from build123d import *

# Parameters (mm, degrees)
SKETCH7_R           = 1.5
SKETCH7_R_2         = 3.5
SKETCH7_R_3         = 1
BOSS_EXTRUDE1_DEPTH = 3.5
FILLET8_R           = 10
FILLET14_R          = 1
FILLET15_R          = 1
FILLET16_R          = 1


with BuildPart() as part:
    # Sketch7 → Boss-Extrude1 (new body)
    with BuildSketch(Plane.XY):
        with BuildLine():
            Line((81.96877708, 8.838834765), (95.403805922, -4.596194078))
            ThreePointArc((95.403805922, -4.596194078), (104.596194078, -4.596194078), (104.596194078, 4.596194078))
            Line((104.596194078, 4.596194078), (91.161165235, 18.03122292))
            Line((91.161165235, 18.03122292), (93.636038969, 20.506096654))
            Line((93.636038969, 20.506096654), (44.142135624, 70))
            Line((44.142135624, 70), (6, 70))
            Line((6, 70), (3.453220204, 85.420324662))
            ThreePointArc((3.453220204, 85.420324662), (0, 88.35), (-3.453220204, 85.420324662))
            Line((-3.453220204, 85.420324662), (-6, 70))
            Line((-6, 70), (-44.142135624, 70))
            Line((-44.142135624, 70), (-63.587572106, 50.554563517))
            Line((-63.587572106, 50.554563517), (-49.445436483, 36.412427894))
            Line((-49.445436483, 36.412427894), (-35.857864376, 50))
            Line((-35.857864376, 50), (35.857864376, 50))
            Line((35.857864376, 50), (79.493903346, 6.363961031))
            Line((79.493903346, 6.363961031), (81.96877708, 8.838834765))
        make_face()
        with Locations((0, 84.85)):
            Circle(SKETCH7_R, mode=Mode.SUBTRACT)
        with Locations((0, 60)):
            Circle(SKETCH7_R, mode=Mode.SUBTRACT)
        with Locations((100, 0)):
            Circle(SKETCH7_R_2, mode=Mode.SUBTRACT)
        with Locations((86.564971157, 20.506096654)):
            Circle(SKETCH7_R_3, mode=Mode.SUBTRACT)
        with Locations((79.493903346, 13.435028843)):
            Circle(SKETCH7_R_3, mode=Mode.SUBTRACT)
        with Locations((-50, 50)):
            Circle(SKETCH7_R, mode=Mode.SUBTRACT)
    extrude(amount=BOSS_EXTRUDE1_DEPTH)

    # Fillet8
    fillet8_edges = [part.edges().sort_by_distance(p)[0] for p in [
        (-44.142135624, 70, 1.75),
        (44.142135624, 70, 1.75),
    ]]
    fillet(fillet8_edges, radius=FILLET8_R)

    # Fillet14
    fillet14_edges = [part.edges().sort_by_distance(p)[0] for p in [
        (93.636038969, 20.506096654, 1.75),
        (91.161165235, 18.03122292, 1.75),
    ]]
    fillet(fillet14_edges, radius=FILLET14_R)

    # Fillet15
    fillet15_edges = [part.edges().sort_by_distance(p)[0] for p in [
        (-49.445436483, 36.412427894, 1.75),
        (-63.587572106, 50.554563517, 1.75),
        (81.96877708, 8.838834765, 1.75),
        (79.493903346, 6.363961031, 1.75),
    ]]
    fillet(fillet15_edges, radius=FILLET15_R)

    # Fillet16
    fillet16_edges = [part.edges().sort_by_distance(p)[0] for p in [
        (-6, 70, 1.75),
        (6, 70, 1.75),
    ]]
    fillet(fillet16_edges, radius=FILLET16_R)


solid = part.part
Here's how the part is built. I have some questions about the finished solid (model axes, mm). A direction names the side the tool comes from. Round coordinates to 2 decimals unless told otherwise and drop trailing zeros. Write each loop counter-clockwise with the first axis right and the second up, starting at its lowest first coordinate (ties: lowest second). Pieces come first, ordered by that corner, then holes. Notation, with made-up numbers: (8.5, 47) -> (60.5, 47) arc R24 cw to (60.5, 57) -> close; hole circle Ø5 at (47.25, -39.75). An arc over 180 degrees is marked (long way). One line per item, written item: value.
1) Suppose I cut it at A-A on z = 2.95. Give the number of separate pieces and of enclosed holes in the cut face, plus the area to 3 significant figures.
Filled sheet:
separate pieces: 1
enclosed holes: 6
area: 3,790 mm2
2) If I drill on line 1 (Y direction, x = 0, z = 0.9); line 2 (Y direction, x = 22.5, z = 0.6); line 3 (Y direction, x = 100, z = 1.4), over which ranges is the centre line in solid material (lowest first)? Write a range as [from, to].
Filled sheet:
line 1: y = [50, 58.5], [61.5, 83.35], [86.35, 88.35]
line 2: y = [50, 70]
line 3: y = [-6.5, -3.5], [3.5, 9.19]
3) I'm going to push flat-ended pins straight in: pin 1 Ø1.5 at (y, z) = (43.5, 0.5) entering from +X; pin 2 Ø1.8 at (x, y) = (0, 60) entering from -Z; pin 3 Ø1 at (x, z) = (78, 1.5) entering from -Y; pin 4 Ø1 at (x, z) = (15.5, 2) entering from -Y. Where does each tip first touch, or does it pass through?
Filled sheet:
pin 1: stops at x = 71.39
pin 2: passes through
pin 3: stops at y = 7.36
pin 4: stops at y = 50
4) Suppose I cut it at D-D on y = 74. List the corners of the cut face in (x, z) for me, plus the area to 3 significant figures.
Filled sheet:
outline: (-5.34, 0) -> (5.34, 0) -> (5.34, 3.5) -> (-5.34, 3.5) -> close
area: 37.4 mm2
5) Suppose I cut it at B-B on y = 0. List the corners of the cut face in (x, z) for me.
Filled sheet:
outline: (90.81, 0) -> (96.5, 0) -> (96.5, 3.5) -> (90.81, 3.5) -> close; (103.5, 0) -> (106.5, 0) -> (106.5, 3.5) -> (103.5, 3.5) -> close
6) For faces 4 (the face through (-23, 70, 2)), 5 (the face through (-1, 50, 2)), 6 (the face through (24, 70, 2)), which set-ups out of +Z, -Z, +X, -X, +Y, -Y let a thin tool reach every point of the face, with its end or its side?
Filled sheet:
face 4: +Z, -Z, -X, +Y
face 5: +Z, -Z, -Y
face 6: +Z, -Z, +X, +Y
7) We'd pull the mould along Y, two halves only. Please class faces 1 (the face through (57.02, 28.84, 1.73)), 2 (the face through (-0.195, 61.487, 1.726)), 3 (the face through (104.49, -4.7, 1.73)): released by +Y, released by -Y, zero draft, split by the parting line, or undercut.
Filled sheet:
face 1: released by -Y
face 2: undercut
face 3: split by the parting line
8) Suppose I cut it at C-C on x = -14. List the corners of the cut face in (y, z) for me.
Filled sheet:
outline: (50, 0) -> (70, 0) -> (70, 3.5) -> (50, 3.5) -> close
